Work out the finished part from the listing and answer in its coordinate system (mm). Give positions to 0.01 mm unless a question says otherwise; leave off trailing zeros. Loops run counter-clockwise (first coordinate to the right, second up) from the corner with the lowest first, then second, coordinate; pieces in that order, holes last. Notation, with made-up numbers: M 83,-14 L 123,-14 A10 cw 123,-6 Z; hole C -17.75,10 d4. An arc over 180 degrees is marked long. Answer as a JSON object with one key per item and string values. Group by question number.
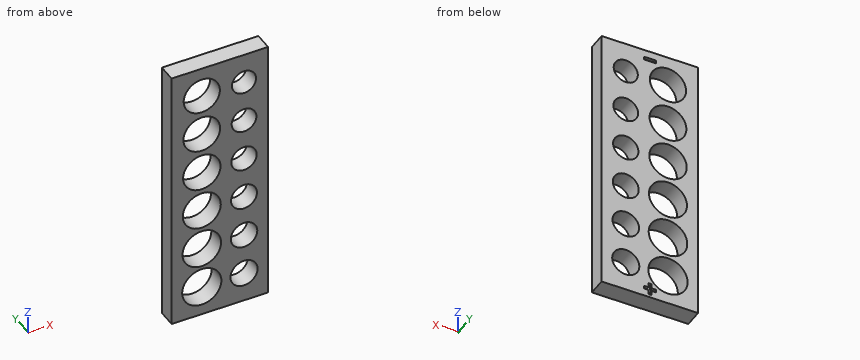
```python
from build123d import *

# Parameters (mm, degrees)
SKETCH1_W           = 16
SKETCH1_H           = 45
SKETCH1_R           = 3
SKETCH1_R_2         = 3.05
SKETCH1_R_3         = 3.1
SKETCH1_R_4         = 3.15
SKETCH1_R_5         = 3.2
SKETCH1_R_6         = 3.25
SKETCH1_R_7         = 2.25
SKETCH1_R_8         = 2.2
SKETCH1_R_9         = 2.15
SKETCH1_R_10        = 2.1
SKETCH1_R_11        = 2.05
SKETCH1_R_12        = 2
BOSS_EXTRUDE1_DEPTH = 3
SKETCH2_W           = 2
SKETCH2_H           = 0.5
CUT_EXTRUDE1_DEPTH  = 0.5


with BuildPart() as part:
    # Sketch1 → Boss-Extrude1 (new body)
    with BuildSketch(Plane(origin=(0, 0, 0), x_dir=(1, 0, 0), z_dir=(0, 1, 0))):
        with Locations((8, 22.5)):
            Rectangle(SKETCH1_W, SKETCH1_H)
        with Locations((5, 5)):
            Circle(SKETCH1_R, mode=Mode.SUBTRACT)
        with Locations((5, 12)):
            Circle(SKETCH1_R_2, mode=Mode.SUBTRACT)
        with Locations((5, 19)):
            Circle(SKETCH1_R_3, mode=Mode.SUBTRACT)
        with Locations((5, 26)):
            Circle(SKETCH1_R_4, mode=Mode.SUBTRACT)
        with Locations((5, 33)):
            Circle(SKETCH1_R_5, mode=Mode.SUBTRACT)
        with Locations((5, 40)):
            Circle(SKETCH1_R_6, mode=Mode.SUBTRACT)
        with Locations((12, 40)):
            Circle(SKETCH1_R_7, mode=Mode.SUBTRACT)
        with Locations((12, 33)):
            Circle(SKETCH1_R_8, mode=Mode.SUBTRACT)
        with Locations((12, 26)):
            Circle(SKETCH1_R_9, mode=Mode.SUBTRACT)
        with Locations((12, 19)):
            Circle(SKETCH1_R_10, mode=Mode.SUBTRACT)
        with Locations((12, 12)):
            Circle(SKETCH1_R_11, mode=Mode.SUBTRACT)
        with Locations((12, 5)):
            Circle(SKETCH1_R_12, mode=Mode.SUBTRACT)
    extrude(amount=BOSS_EXTRUDE1_DEPTH)

    # Sketch2 → Cut-Extrude1 (cut)
    with BuildSketch(Plane(origin=(0, 3, 0), x_dir=(1, 0, 0), z_dir=(0, 1, 0))):
        Polygon((7.75, 43.75), (7.75, 44.5), (8.25, 44.5), (8.25, 43.75), (9, 43.75), (9, 43.25), (8.25, 43.25), (8.25, 42.5), (7.75, 42.5), (7.75, 43.25), (7, 43.25), (7, 43.75), align=None)
        with Locations((8, 1.5)):
            Rectangle(SKETCH2_W, SKETCH2_H)
    extrude(amount=-CUT_EXTRUDE1_DEPTH, mode=Mode.SUBTRACT)


solid = part.part
```
Item 1: A cutting plane is placed at C-C (y = 2.05). Give the number of separate pieces and of enclosed holes in the cut face, and give its area (3 significant figures).
Item 2: A cutting plane is placed at D-D (z = -33). Determine the outline of the cut face in (x, y), and give its area (3 significant figures).
Item 3: Find the intervals of material crossed by probe 1 along X at (y, z) = (2.15, -26); probe 2 along X at (y, z) = (2.1, -12); probe 3 along X at (y, z) = (1.9, -2.5), in increasing order. Write a range as [from, to].
Item 4: A cutting plane is placed at A-A (z = -19). Determine the outline of the cut face in (x, y).
Item 5: Given pin 1 Ø3.5 at (x, z) = (5, -12) entering from +Y, flat-ended and moving along its own axis, determine where the tip first touches the part or whether it passes through.
Item 6: A cutting plane is placed at B-B (x = 12). Determine the outline of the cut face in (y, z).
The answers:
{
 "1": {"separate pieces": "1", "enclosed holes": "12", "area": "451 mm^2"},
 "2": {"outline": "M 0,0 L 1.8,0 L 1.8,3 L 0,3 Z; M 8.2,0 L 9.8,0 L 9.8,3 L 8.2,3 Z; M 14.2,0 L 16,0 L 16,3 L 14.2,3 Z", "area": "15.6 mm^2"},
 "3": {"probe 1": "x = [0, 1.85], [8.15, 9.85], [14.15, 16]", "probe 2": "x = [0, 1.95], [8.05, 9.95], [14.05, 16]", "probe 3": "x = [0, 3.34], [6.66, 16]"},
 "4": {"outline": "M 0,0 L 1.9,0 L 1.9,3 L 0,3 Z; M 8.1,0 L 9.9,0 L 9.9,3 L 8.1,3 Z; M 14.1,0 L 16,0 L 16,3 L 14.1,3 Z"},
 "5": {"pin 1": "passes through"},
 "6": {"outline": "M 0,-45 L 3,-45 L 3,-42.25 L 0,-42.25 Z; M 0,-37.75 L 3,-37.75 L 3,-35.2 L 0,-35.2 Z; M 0,-30.8 L 3,-30.8 L 3,-28.15 L 0,-28.15 Z; M 0,-23.85 L 3,-23.85 L 3,-21.1 L 0,-21.1 Z; M 0,-16.9 L 3,-16.9 L 3,-14.05 L 0,-14.05 Z; M 0,-9.95 L 3,-9.95 L 3,-7 L 0,-7 Z; M 0,-3 L 3,-3 L 3,0 L 0,0 Z"}
}
